from build123d import *

# Parameters (mm, degrees)
F0_W     = 38
F0_H     = 19
F0_R     = 1.5
F1_DEPTH = 3
F2_W     = 2
F2_H     = 2
F3_DEPTH = 38
F5_DEPTH = 5
F6_DEPTH = 11
F8_DEPTH = 1.5


with BuildPart() as f1:
    # F0 (on Top) → F1 (new body)
    with BuildSketch(Plane.XY):
        Rectangle(F0_W, F0_H)
        with Locations((-10.5, -3)):
            Circle(F0_R, mode=Mode.SUBTRACT)
        with Locations((10.5, -3)):
            Circle(F0_R, mode=Mode.SUBTRACT)
    extrude(amount=F1_DEPTH)

    # F2 (on face) → F3 (join)
    with BuildSketch(Plane.YZ.offset(19)):
        with Locations((-8.5, -1)):
            Rectangle(F2_W, F2_H)
    extrude(amount=-F3_DEPTH)

    # F4 (on face) → F5 (join)
    with BuildSketch(Plane(origin=(0, 9.5, 0), x_dir=(-1, 0, 0), z_dir=(0, 1, 0))):
        with BuildLine():
            Line((19, 3), (6, 33))
            ThreePointArc((6, 33), (0, 27), (-6, 33))
            Line((-6, 33), (-19, 3))
            Line((-19, 3), (19, 3))
        make_face()
    extrude(amount=-F5_DEPTH)

    # F4 (on face) → F6 (join)
    with BuildSketch(Plane(origin=(0, 9.5, 0), x_dir=(-1, 0, 0), z_dir=(0, 1, 0))):
        with BuildLine():
            ThreePointArc((-2.5, 33), (0, 35.5), (2.5, 33))
            Line((2.5, 33), (6, 33))
            ThreePointArc((6, 33), (0, 39), (-6, 33))
            Line((-6, 33), (-2.5, 33))
        make_face()
        with BuildLine():
            Line((6, 33), (2.5, 33))
            ThreePointArc((2.5, 33), (0, 30.5), (-2.5, 33))
            Line((-2.5, 33), (-6, 33))
            ThreePointArc((-6, 33), (0, 27), (6, 33))
        make_face()
    extrude(amount=-F6_DEPTH)

    # F7 (on Right) → F8 (join, symmetric)
    with BuildSketch(Plane.YZ):
        Polygon((-1.5, 27.080068), (-9.5, 3), (4.5, 3), (4.5, 27.080068), align=None)
    extrude(amount=F8_DEPTH, both=True)


solid = f1.part
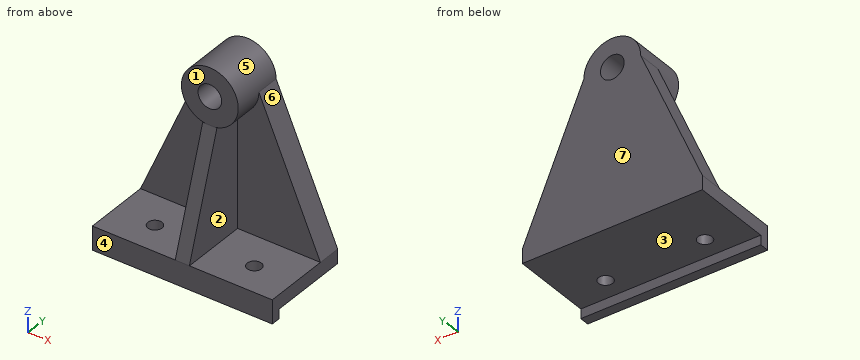
Here's how the part is built. I have some questions about the finished solid (model axes, mm). Face numbers are marked on the shaded views. A direction names the side the tool comes from. Coordinates: 2 decimals unless noted, no trailing zeros. Order: outer loops, then holes, each group sorted by start corner. A loop starts at its lowest first (then second) coordinate and runs counter-clockwise, first axis right, second up. Notation, with made-up numbers: (54, 84) -> (78, 84) arc R24 ccw to (78, 111) -> close; hole circle Ø3 at (-27.75, 50). An arc over 180 degrees is marked (long way). Answer in a Markdown table with one row per item.
(1) I want a section at B-B on x = 0. List the corners of the cut face in (y, z) for me, then the cut area to 3 significant figures.
Answer key:
| item | result |
|---|---|
| outline | (-9.5, -2) -> (-7.5, -2) -> (-7.5, 0) -> (9.5, 0) -> (9.5, 30.5) -> (-1.5, 30.5) -> (-1.5, 27.08) -> (-9.5, 3) -> close; (-1.5, 35.5) -> (9.5, 35.5) -> (9.5, 39) -> (-1.5, 39) -> close |
| area | 498 mm^2 |
(2) I want a section at D-D on z = 3.5. List the corners of the cut face in (x, y) for me.
Answer key:
| item | result |
|---|---|
| outline | (-18.78, 4.5) -> (-1.5, 4.5) -> (-1.5, -9.33) -> (1.5, -9.33) -> (1.5, 4.5) -> (18.78, 4.5) -> (18.78, 9.5) -> (-18.78, 9.5) -> close |
(3) I want a section at A-A on y = 7.75. List the corners of the cut face in (x, z) for me, then the cut area to 3 significant figures.
Answer key:
| item | result |
|---|---|
| outline | (-19, 0) -> (19, 0) -> (19, 3) -> (6, 33) arc R6 ccw to (-6, 33) -> (-19, 3) -> close; hole circle Ø5 at (0, 33) |
| area | 901 mm^2 |
(4) Please list where these lines run through material, in increasing order: probe 1 along Y at (x, z) = (10.5, 1.65); probe 2 along X at (y, z) = (7, 33); probe 3 along Y at (x, z) = (-4, 30.5).
Answer key:
| item | result |
|---|---|
| probe 1 | -9.5 to -4.5, -1.5 to 9.5 |
| probe 2 | -6 to -2.5, 2.5 to 6 |
| probe 3 | -1.5 to 9.5 |
(5) Will these pins go through, and if not, where does the flat tip stop? pin 1 Ø6.5 at (x, z) = (0, 33) entering from -Y; pin 2 Ø10 at (x, y) = (-14, 5.5) entering from +Z; pin 3 Ø2 at (x, y) = (-7, -3) entering from -Z; pin 4 Ø4 at (y, z) = (-3.5, 4.5) entering from -X.
Answer key:
| item | result |
|---|---|
| pin 1 | y = -1.5 |
| pin 2 | z = 26.08 |
| pin 3 | z = 0 |
| pin 4 | x = -19 |
(6) On a 3-axis mill with a long thin cutter (end or side, diameter ignored), from which of +Z, -Z, +X, -X, +Y, -Y can I reach the whole of each face in a straight line? I mean the marked faces 1, 2, 3 and 4. Say none if no direction works.
Answer key:
| item | result |
|---|---|
| face 1 | +Z, +X, -X, -Y |
| face 2 | +X, -Y |
| face 3 | -Z, +X, -X, +Y |
| face 4 | +Z, -Z, +X, -X, -Y |
(7) Thinking about a two-plate mould opening in Z: for the marked faces 5, 6 and 7, which applies, +Z half, -Z half, draft (parallel to the pull), parting line (faces both ways), or undercut?
Answer key:
| item | result |
|---|---|
| face 5 | undercut |
| face 6 | +Z half |
| face 7 | draft |
(8) I want a section at C-C on y = -3. List the corners of the cut face in (x, z) for me.
Answer key:
| item | result |
|---|---|
| outline | (-19, 0) -> (-12, 0) -> (-12, 3) -> (-19, 3) -> close; (-9, 0) -> (9, 0) -> (9, 3) -> (1.5, 3) -> (1.5, 22.57) -> (-1.5, 22.57) -> (-1.5, 3) -> (-9, 3) -> close; (12, 0) -> (19, 0) -> (19, 3) -> (12, 3) -> close |
